from build123d import *

# Parameters (mm, degrees)
SKETCH1_R           = 2.9337
BOSS_EXTRUDE1_DEPTH = 25.4


with BuildPart() as part:
    # Sketch1 → Boss-Extrude1 (new body)
    with BuildSketch(Plane.XY):
        with BuildLine():
            Line((-4.705511314, -4.549815329), (-3.666174209, -6.35))
            Line((-3.666174209, -6.35), (-1.5875, -6.35))
            ThreePointArc((-1.5875, -6.35), (0, -4.7625), (1.5875, -6.35))
            Line((1.5875, -6.35), (3.666174209, -6.35))
            Line((3.666174209, -6.35), (4.705511314, -4.549815329))
            ThreePointArc((4.705511314, -4.549815329), (4.124445986, -2.38125), (6.293011314, -1.800184671))
            Line((6.293011314, -1.800184671), (7.332348419, 0))
            Line((7.332348419, 0), (6.293011314, 1.800184671))
            ThreePointArc((6.293011314, 1.800184671), (4.124445986, 2.38125), (4.705511314, 4.549815329))
            Line((4.705511314, 4.549815329), (3.666174209, 6.35))
            Line((3.666174209, 6.35), (1.5875, 6.35))
            ThreePointArc((1.5875, 6.35), (0, 4.7625), (-1.5875, 6.35))
            Line((-1.5875, 6.35), (-3.666174209, 6.35))
            Line((-3.666174209, 6.35), (-4.705511314, 4.549815329))
            ThreePointArc((-4.705511314, 4.549815329), (-4.124445986, 2.38125), (-6.293011314, 1.800184671))
            Line((-6.293011314, 1.800184671), (-7.332348419, 0))
            Line((-7.332348419, 0), (-6.293011314, -1.800184671))
            ThreePointArc((-6.293011314, -1.800184671), (-4.124445986, -2.38125), (-4.705511314, -4.549815329))
        make_face()
        Circle(SKETCH1_R, mode=Mode.SUBTRACT)
    extrude(amount=-BOSS_EXTRUDE1_DEPTH)


solid = part.part
The listing builds one solid part. Answer for the finished solid, in the listing's coordinates (mm). Round coordinates to 2 decimals unless told otherwise and drop trailing zeros. Order: outer loops, then holes, each group sorted by start corner. A loop starts at its lowest first (then second) coordinate and runs counter-clockwise, first axis right, second up. Notation, with made-up numbers: (-29, 39) -> (1, 39) arc R28 cw to (1, 62) -> close; hole circle Ø10 at (27.25, 4). An arc over 180 degrees is marked (long way). Put each result on its own line as item: value.
Q1. Consider line 1 along Y through (x, z) = (0, -10.25); line 2 along Y through (x, z) = (-0.75, -4.25); line 3 along X through (y, z) = (-2, -2.5). Determine where each line is inside the solid, lowest interval first.
Results list:
line 1: -4.76 to -2.93, 2.93 to 4.76
line 2: -4.95 to -2.84, 2.84 to 4.95
line 3: -4.43 to -2.15, 2.15 to 4.43
Q2. Section B-B, the plane x = 0 is taken. Write down the section's boundary in (y, z), and give its area (3 significant figures).
Results list:
outline: (-4.76, -25.4) -> (-2.93, -25.4) -> (-2.93, 0) -> (-4.76, 0) -> close; (2.93, -25.4) -> (4.76, -25.4) -> (4.76, 0) -> (2.93, 0) -> close
area: 92.9 mm^2
Q3. Each of these flat-tipped pins is pushed along its axis until it touches: P1, Ø3.5, axis at x = 0, y = 0, coming from the +Z side; P2, Ø1, axis at y = 4.5, z = -20.5, coming from the +X side; P3, Ø5, axis at y = -1, z = -21.5, coming from the -X side; P4, Ø1, axis at x = -5, z = -18.5, coming from the +Y side. Where does it stop, or does it pass through?
Results list:
P1: through
P2: x = 4.71
P3: x = -7.33
P4: y = 4.91
Q4. Section D-D, the plane x = -5 is taken. Write down the section's boundary in (y, z).
Results list:
outline: (-1.67, -25.4) -> (1.67, -25.4) -> (1.67, 0) -> (-1.67, 0) -> close
Q5. Section C-C, the plane y = 0.75 is taken. Write down the section's boundary in (x, z).
Results list:
outline: (-6.9, -25.4) -> (-2.84, -25.4) -> (-2.84, 0) -> (-6.9, 0) -> close; (2.84, -25.4) -> (6.9, -25.4) -> (6.9, 0) -> (2.84, 0) -> close
Q6. Determine the mould class of faces 1 (the flat face through (3.2, 0.1, -25.4)), 2 (the flat face through (-4.19, -5.44, -12.52)), 3 (the cylindrical face through (-0.636, -2.864, -12.522)) for opening direction X: pulls with the +X half, pulls with the -X half, needs draft (parallel to the pull), parting line crosses it, or undercut.
Results list:
face 1: needs draft
face 2: pulls with the -X half
face 3: undercut
